The model under review builds one solid part; all positions refer to its coordinate system, in mm. Face numbers are marked on the shaded views. A direction names the side the tool comes from. Round coordinates to 2 decimals unless told otherwise and drop trailing zeros. Loops run counter-clockwise (first coordinate to the right, second up) from the corner with the lowest first, then second, coordinate; pieces in that order, holes last. Notation, with made-up numbers: M 10,-29.75 L 37,-29.75 A28 ccw 37,1.25 Z; hole C -28,78 d10. An arc over 180 degrees is marked long. Use a Markdown table: item, result. Add a question column.
```python
from build123d import *

# Parameters (mm, degrees)
F1_DEPTH = 7.5
F2_R     = 12.5
F2_R_2   = 2.75
F3_DEPTH = 15
F4_SIZE  = 3
F5_SIZE  = 1
F6_W     = 31
F6_H     = 8.371188
F7_DEPTH = 5


with BuildPart() as f1:
    # F0 (on Front) → F1 (new body, symmetric)
    with BuildSketch(Plane.XZ):
        Polygon((17, 11), (17, 21.5), (-17, 21.5), (-17, 11), (-30, 11), (-30, -21.5), (30, -21.5), (30, 11), align=None)
    extrude(amount=F1_DEPTH, both=True)

    # F2 (on face) → F3 (cut)
    with BuildSketch(Plane.XZ.offset(7.5)):
        with Locations((0, 3.5)):
            Circle(F2_R)
        with Locations((-23, 3.5)):
            Circle(F2_R_2)
        with Locations((23, 3.5)):
            Circle(F2_R_2)
        with Locations((-23, -14.5)):
            Circle(F2_R_2)
        with Locations((23, -14.5)):
            Circle(F2_R_2)
    extrude(amount=-F3_DEPTH, mode=Mode.SUBTRACT)

    # F4
    f4_edges = [f1.edges().sort_by_distance(p)[0] for p in [
        (17, 0, 21.5),
        (-17, 0, 21.5),
    ]]
    chamfer(f4_edges, length=F4_SIZE)

    # F5
    f5_edges = [f1.edges().sort_by_distance(p)[0] for p in [
        (-30, 0, 11),
        (30, 0, 11),
    ]]
    chamfer(f5_edges, length=F5_SIZE)

    # F6 (on face) → F7 (cut)
    with BuildSketch(Plane.XZ.offset(7.5)):
        Polygon((17, -13.5), (17, 20.5), (15.5, 20.5), (-15.5, 20.5), (-17, 20.5), (-17, -13.5), align=None)
        with Locations((0, 24.685594)):
            Rectangle(F6_W, F6_H)
    extrude(amount=-F7_DEPTH, mode=Mode.SUBTRACT)


solid = f1.part
```
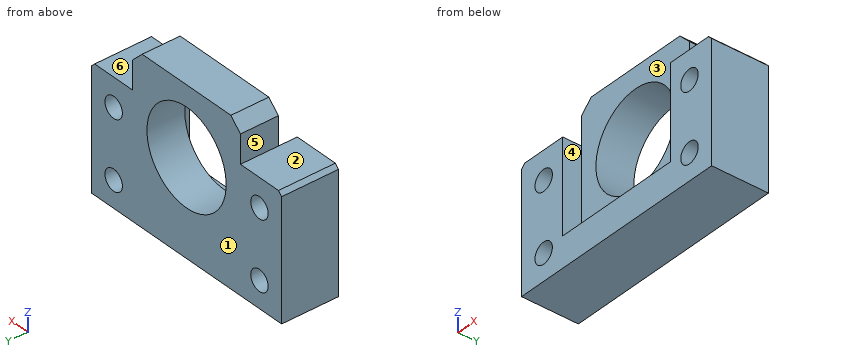
(1) Consider section D-D, the plane z = 3.5. Give the boundary of the cut face in (x, y), then the cut area to 3 significant figures.
(2) Draft analysis for pull direction X (two halves, no side actions). For the marked faces 4, 5 and 6, state which applies: released by +X, released by -X, zero draft, split by the parting line, or undercut.
(3) Consider section A-A, the plane y = -4.25. Give the boundary of the cut face in (x, z).
(4) Insertion check: pin 1 Ø3 at (x, y) = (-23.5, -4) entering from +Z; pin 2 Ø6 at (y, z) = (1.5, 13.5) entering from +X; pin 3 Ø1.5 at (x, y) = (-1, -5) entering from +Z. Each pin has a flat end and moves straight along its axis. Give the tip position at first contact, or say it passes through.
(5) Consider section C-C, the plane z = -14.5. Give the boundary of the cut face in (x, y).
(6) To check wall thickness, follow probe 1 along Z at (x, y) = (-23, -4); probe 2 along Z at (x, y) = (0, 3); probe 3 along Z at (x, y) = (-21, -1.75). State the ranges of each line that lie inside material, in increasing order.
(7) Consider section B-B, the plane x = 10. Give the boundary of the cut face in (y, z).
(8) For the marked faces 1, 2 and 3, list the 3-axis set-ups (+Z, -Z, +X, -X, +Y, -Y) from which the entire face can be reached by the end or side of a thin tool; tool diameter is ignored.
Found:
| question | item | result |
|---|---|---|
| 1 | outline | M -30,-7.5 L -25.75,-7.5 L -25.75,7.5 L -30,7.5 Z; M -20.25,-7.5 L -17,-7.5 L -17,-2.5 L -12.5,-2.5 L -12.5,7.5 L -20.25,7.5 Z; M 12.5,-2.5 L 17,-2.5 L 17,-7.5 L 20.25,-7.5 L 20.25,7.5 L 12.5,7.5 Z; M 25.75,-7.5 L 30,-7.5 L 30,7.5 L 25.75,7.5 Z |
| 1 | area | 315 mm^2 |
| 2 | face 4 | undercut |
| 2 | face 5 | released by -X |
| 2 | face 6 | zero draft |
| 3 | outline | M -30,-21.5 L 30,-21.5 L 30,10 L 29,11 L 17,11 L 17,-13.5 L -17,-13.5 L -17,11 L -29,11 L -30,10 Z; hole C -23,-14.5 d5.5; hole C -23,3.5 d5.5; hole C 23,-14.5 d5.5; hole C 23,3.5 d5.5 |
| 4 | pin 1 | stops at z = 11 |
| 4 | pin 2 | stops at x = 29.5 |
| 4 | pin 3 | stops at z = -13.5 |
| 5 | outline | M -30,-7.5 L -25.75,-7.5 L -25.75,7.5 L -30,7.5 Z; M -20.25,-7.5 L 20.25,-7.5 L 20.25,7.5 L -20.25,7.5 Z; M 25.75,-7.5 L 30,-7.5 L 30,7.5 L 25.75,7.5 Z |
| 6 | probe 1 | z = -21.5 to -17.25, -11.75 to 0.75, 6.25 to 11 |
| 6 | probe 2 | z = -21.5 to -9, 16 to 21.5 |
| 6 | probe 3 | z = -21.5 to -16.39, -12.61 to 1.61, 5.39 to 11 |
| 7 | outline | M -7.5,-21.5 L 7.5,-21.5 L 7.5,-4 L -2.5,-4 L -2.5,-13.5 L -7.5,-13.5 Z; M -2.5,11 L 7.5,11 L 7.5,21.5 L -2.5,21.5 Z |
| 8 | face 1 | +Z, -Z, +X, -X, +Y |
| 8 | face 2 | +Z, -X, +Y, -Y |
| 8 | face 3 | +Z, -Y |
